Input: part model. Units: mm. Frame: model coordinates. A direction names the side the tool comes from. Coordinates: 2 decimals unless noted, no trailing zeros. Order: outer loops, then holes, each group sorted by start corner. A loop starts at its lowest first (then second) coordinate and runs counter-clockwise, first axis right, second up.
from build123d import *

# Parameters (mm, degrees)
BOSS_EXTRUDE1_DEPTH = 200
SHELL3_T            = -5
CUT_EXTRUDE1_DEPTH  = 195
BOSS_EXTRUDE2_DEPTH = 200
BOSS_EXTRUDE3_DEPTH = 200
SKETCH5_R           = 1.998576913
CUT_EXTRUDE2_DEPTH  = 210


with BuildPart() as part:
    # Sketch1 → Boss-Extrude1 (new body)
    with BuildSketch(Plane(origin=(0, 0, 0), x_dir=(1, 0, 0), z_dir=(0, 1, 0))):
        with BuildLine():
            Line((0, 0), (200, 0))
            Line((200, 0), (200, -70.8103799))
            ThreePointArc((200, -70.8103799), (196.311654881, -82.383189198), (186.607008495, -89.687547027))
            Line((186.607008495, -89.687547027), (106.607008495, -117.687547027))
            ThreePointArc((106.607008495, -117.687547027), (100, -118.8103799), (93.392991505, -117.687547027))
            Line((93.392991505, -117.687547027), (13.392991505, -89.687547027))
            ThreePointArc((13.392991505, -89.687547027), (3.688345119, -82.383189198), (0, -70.8103799))
            Line((0, -70.8103799), (0, 0))
        make_face()
    extrude(amount=BOSS_EXTRUDE1_DEPTH)

    # Shell3
    shell3_openings = [part.faces().sort_by_distance(p)[0] for p in [
        (100, 200, 51.617363214),
        (100, 0, 51.617363214),
    ]]
    offset(amount=SHELL3_T, openings=shell3_openings, kind=Kind.INTERSECTION)

    # Sketch2 → Cut-Extrude1 (cut)
    with BuildSketch(Plane(origin=(0, 0, 0), x_dir=(1, 0, 0), z_dir=(0, 1, 0))):
        Polygon((195, 0), (187.458653408, 0), (12.307944586, 0), (5, 0), (5, -3), (11, -3), (11, -5), (189, -5), (189, -3), (195, -3), align=None)
    extrude(amount=CUT_EXTRUDE1_DEPTH, mode=Mode.SUBTRACT)

    # Sketch3 → Boss-Extrude2 (add)
    with BuildSketch(Plane(origin=(0, 0, 0), x_dir=(1, 0, 0), z_dir=(0, 1, 0))):
        Polygon((5, -5), (5, -11), (11, -5), align=None)
        Polygon((195, -5), (195, -11), (189, -5), align=None)
    extrude(amount=BOSS_EXTRUDE2_DEPTH)

    # Sketch4 → Boss-Extrude3 (add)
    with BuildSketch(Plane(origin=(0, 0, 0), x_dir=(1, 0, 0), z_dir=(0, 1, 0))):
        Polygon((5, -70.8103799), (17, -70.8103799), (17, -85.652594975), (13.392991505, -89.687547027), (0, -70.8103799), align=None)
        Polygon((195, -70.8103799), (183, -70.8103799), (183, -85.652594975), (186.607008495, -89.687547027), (200, -70.8103799), align=None)
    extrude(amount=BOSS_EXTRUDE3_DEPTH)

    # Sketch5 → Cut-Extrude2 (cut)
    with BuildSketch(Plane(origin=(0, 0, 0), x_dir=(1, 0, 0), z_dir=(0, 1, 0))):
        with Locations(Location((9.743456049, -76.677329473, 0), (0, 0, 90))):
            Circle(SKETCH5_R)
        with Locations(Location((190.256543951, -76.677329473, 0), (0, 0, 90))):
            Circle(SKETCH5_R)
    extrude(amount=CUT_EXTRUDE2_DEPTH, mode=Mode.SUBTRACT)


solid = part.part
Item 1: Cut plane B-B on x = 50. Return loops of the section in (y, z), then the cut area to 3 significant figures.
Response values:
outline: (0, 97.2) - (200, 97.2) - (200, 102.5) - (0, 102.5) - close; (195, 0) - (200, 0) - (200, 5) - (195, 5) - close
area: 1,080 mm2
Item 2: Access query for faces 1 (the face through (195, 99, 40)), 2 (the face through (192, 96, 3)), 3 (the face through (123, 0, 108)). Directions: +Z, -Z, +X, -X, +Y, -Y. A direction counts if a zero-diameter tool reaches every point of the face in a straight line with its end or side. Return the directions, or none.
Response values:
face 1: +Y, -Y
face 2: -Z, -Y
face 3: +Z, -Z, +X, -X, -Y
Item 3: Ray query, probe 1 along X at (y, z) = (49, 15); probe 2 along X at (y, z) = (10, 81); probe 3 along Z at (x, y) = (25.5, 170) (3 decimals). Return the intervals inside material, ascending.
Response values:
probe 1: x = 0 to 5, 195 to 200
probe 2: x = 2.79 to 17, 183 to 197.21
probe 3: z = 88.628 to 93.925
Item 4: Cut plane C-C on y = 60. Return loops of the section in (x, z), then the cut area to 3 significant figures.
Response values:
outline: (0, 0) - (5, 0) - (5, 3) - (11, 3) - (11, 5) - (5, 11) - (5, 70.81) - (17, 70.81) - (17, 85.65) - (95.04, 112.97) arc R15 cw to (104.96, 112.97) - (183, 85.65) - (183, 70.81) - (195, 70.81) - (195, 11) - (189, 5) - (189, 3) - (195, 3) - (195, 0) - (200, 0) - (200, 70.81) arc R20 ccw to (186.61, 89.69) - (106.61, 117.69) arc R20 ccw to (93.39, 117.69) - (13.39, 89.69) arc R20 ccw to (0, 70.81) - close; hole circle Ø4 at (9.74, 76.68); hole circle Ø4 at (190.26, 76.68)
area: 2,130 mm2
Item 5: Draft query along Z for faces 4 (the face through (147.17, 98.6, 103.49)), 5 (the face through (200, 99, 35)), 6 (the face through (11, 99, 70.81)). Return one class per face: pulls with the +Z half, pulls with the -Z half, needs draft (parallel to the pull), parting line crosses it, or undercut.
Response values:
face 4: pulls with the +Z half
face 5: needs draft
face 6: undercut
Item 6: Cut plane A-A on z = 18.5. Return loops of the section in (x, y).
Response values:
outline: (0, 0) - (5, 0) - (5, 200) - (0, 200) - close; (195, 0) - (200, 0) - (200, 200) - (195, 200) - close
Item 7: Pin query (flat end, axial travel): pin 1 Ø2.5 at (x, z) = (93, 3) entering from -Y; pin 2 Ø4.5 at (y, z) = (115, 77) entering from -X; pin 3 Ø6.5 at (x, y) = (8.5, 55) entering from -Z; pin 4 Ø6.5 at (x, z) = (9.74, 76.68) entering from -Y. Return the tip coordinate at first contact, or that it passes through.
Response values:
pin 1: stops at y = 195
pin 2: stops at x = 0.39
pin 3: stops at z = 3
pin 4: stops at y = 0
